```python
from build123d import *

# Parameters (mm, degrees)
SKETCH1_W           = 20
SKETCH1_H           = 20
SKETCH1_W_2         = 17
SKETCH1_H_2         = 17
BOSS_EXTRUDE1_DEPTH = 40
SKETCH2_R           = 2.125
CUT_EXTRUDE1_DEPTH  = 46.82575695


with BuildPart() as part:
    # Sketch1 → Boss-Extrude1 (new body)
    with BuildSketch(Plane.XY):
        Rectangle(SKETCH1_W, SKETCH1_H)
        Rectangle(SKETCH1_W_2, SKETCH1_H_2, mode=Mode.SUBTRACT)
    extrude(amount=-BOSS_EXTRUDE1_DEPTH)

    # Sketch2 → Cut-Extrude1 (cut, through all)
    with BuildSketch(Plane(origin=(0, 10, 0), x_dir=(1, 0, 0), z_dir=(0, 1, 0))):
        with Locations(Location((0, 10, 0), (0, 0, 270))):
            Circle(SKETCH2_R)
        with Locations((0, 80)):
            Circle(SKETCH2_R)
        with Locations((0, 150)):
            Circle(SKETCH2_R)
    extrude(amount=-CUT_EXTRUDE1_DEPTH, mode=Mode.SUBTRACT)


solid = part.part
```
Can you work these out from the model? Positions are in its coordinate system, mm. A direction names the side the tool comes from. Coordinates: 2 decimals unless noted, no trailing zeros. Loops run counter-clockwise (first coordinate to the right, second up) from the corner with the lowest first, then second, coordinate; pieces in that order, holes last. Notation, with made-up numbers: (-29.75, 8.25) -> (-5.75, 8.25) arc R20 cw to (-5.75, 14.25) -> close; hole circle Ø8 at (6, -3). An arc over 180 degrees is marked (long way). Put each result on its own line as item: value. Start each with the question number.
Q1. If I drill on line 1 (Y direction, x = 3.5, z = -24); line 2 (X direction, y = -9.3, z = -10) (3 decimals), over which ranges is the centre line in solid material (lowest first)? Write a range as [from, to].
Q2. I want a section at B-B (y = 7.25). Write out the boundary of the cut face in (x, z).
Q3. For faces 5 (the face through (8.5, 0, -20)), 6 (the face through (-9, 0, -40)), which set-ups out of +Z, -Z, +X, -X, +Y, -Y let a thin tool reach every point of the face, with its end or its side?
Q4. Thinking about a two-plate mould opening in X: for faces 1 (the face through (10, 0, -20)), 2 (the face through (2.107, -9.24, -10.277)), 3 (the face through (0, 10, -20)), 4 (the face through (0, -8.5, -20)), which applies, pulls with the +X half, pulls with the -X half, needs draft (parallel to the pull), parting line crosses it, or undercut?
Q5. I want a section at A-A (x = 0). Write out the boundary of the cut face in (y, z) (3 decimals), plus the area to 3 significant figures.
Q6. I want a section at D-D (z = -24.5). Write out the boundary of the cut face in (x, y).
Q7. I want a section at C-C (z = -10). Write out the boundary of the cut face in (x, y) (3 decimals), plus the area to 4 significant figures.
Taken from the geometry:
1. line 1: y = [-10, -8.5], [8.5, 10]
1. line 2: x = [-10, -2.125], [2.125, 10]
2. outline: (-10, -40) -> (-8.5, -40) -> (-8.5, 0) -> (-10, 0) -> close; (8.5, -40) -> (10, -40) -> (10, 0) -> (8.5, 0) -> close
3. face 5: +Z, -Z
3. face 6: -Z, +X, -X, +Y, -Y
4. face 1: pulls with the +X half
4. face 2: undercut
4. face 3: needs draft
4. face 4: undercut
5. outline: (-10, -40) -> (-8.5, -40) -> (-8.5, -12.125) -> (-10, -12.125) -> close; (-10, -7.875) -> (-8.5, -7.875) -> (-8.5, 0) -> (-10, 0) -> close; (8.5, -40) -> (10, -40) -> (10, -12.125) -> (8.5, -12.125) -> close; (8.5, -7.875) -> (10, -7.875) -> (10, 0) -> (8.5, 0) -> close
5. area: 107 mm2
6. outline: (-10, -10) -> (10, -10) -> (10, 10) -> (-10, 10) -> close; hole (-8.5, -8.5) -> (8.5, -8.5) -> (8.5, 8.5) -> (-8.5, 8.5) -> close
7. outline: (-10, -10) -> (-2.125, -10) -> (-2.125, -8.5) -> (-8.5, -8.5) -> (-8.5, 8.5) -> (-2.125, 8.5) -> (-2.125, 10) -> (-10, 10) -> close; (2.125, -10) -> (10, -10) -> (10, 10) -> (2.125, 10) -> (2.125, 8.5) -> (8.5, 8.5) -> (8.5, -8.5) -> (2.125, -8.5) -> close
7. area: 98.25 mm2
